Read the model definition and answer for the solid it produces. Units are mm, in the model's axes. A direction names the side the tool comes from. Give positions to 0.01 mm unless a question says otherwise; leave off trailing zeros.
Item 1: A cutting plane is placed at A-A (z = 43). State how many separate pieces and enclosed holes the cut face has, plus the area to 3 significant figures.
Item 2: Given pin 1 Ø1 at (x, z) = (0.5, 168.5) entering from +Y; pin 2 Ø0.6 at (x, z) = (-3, 123.5) entering from +Y, each flat-ended and moving along its own axis, determine where each tip first touches the part or whether it passes through.
Item 3: Which of the six approach directions +Z, -Z, +X, -X, +Y, -Y give full straight-line access (tool end or side, diameter ignored) to faces 1 (the face through (0, 4.5, 148)), 2 (the face through (-10, -6, 148))?
Item 4: Find the intervals of material crossed by line 1 along Y through (x, z) = (2.25, 271.5); line 2 along X through (y, z) = (0, 269.5); line 3 along Y through (x, z) = (2, 285.5), in increasing order.
Item 5: The mould has two halves that part along Y. Classify faces 3 (the face through (0, -8.5, 148)), 4 (the face through (4, 0, 0)), 5 (the face through (0, -10, 148)): +Y half, -Y half, draft (parallel to the pull), parting line (faces both ways), or undercut.
from build123d import *

# Parameters (mm, degrees)
BOSS_EXTRUDE1_DEPTH = 1000
CUT_EXTRUDE1_DEPTH  = 700


with BuildPart() as part:
    # Sketch1 → Boss-Extrude1 (new body)
    with BuildSketch(Plane.XY):
        with BuildLine():
            Line((6, 7.06066017), (3.43933983, 4.5))
            Line((3.43933983, 4.5), (-3.43933983, 4.5))
            Line((-3.43933983, 4.5), (-6, 7.06066017))
            Line((-6, 7.06066017), (-6, 8.5))
            Line((-6, 8.5), (-3, 8.5))
            Line((-3, 8.5), (-3, 9.5))
            Line((-3, 9.5), (-3.5, 9.5))
            Line((-3.5, 9.5), (-3.5, 10))
            Line((-3.5, 10), (-8.5, 10))
            ThreePointArc((-8.5, 10), (-9.56066017, 9.56066017), (-10, 8.5))
            Line((-10, 8.5), (-10, 3.5))
            Line((-10, 3.5), (-9.5, 3.5))
            Line((-9.5, 3.5), (-9.5, 3))
            Line((-9.5, 3), (-8.5, 3))
            Line((-8.5, 3), (-8.5, 6))
            Line((-8.5, 6), (-7.06066017, 6))
            Line((-7.06066017, 6), (-4.5, 3.43933983))
            Line((-4.5, 3.43933983), (-4.5, -3.43933983))
            Line((-4.5, -3.43933983), (-7.06066017, -6))
            Line((-7.06066017, -6), (-8.5, -6))
            Line((-8.5, -6), (-8.5, -3))
            Line((-8.5, -3), (-9.5, -3))
            Line((-9.5, -3), (-9.5, -3.5))
            Line((-9.5, -3.5), (-10, -3.5))
            Line((-10, -3.5), (-10, -8.5))
            ThreePointArc((-10, -8.5), (-9.56066017, -9.56066017), (-8.5, -10))
            Line((-8.5, -10), (8.5, -10))
            ThreePointArc((8.5, -10), (9.56066017, -9.56066017), (10, -8.5))
            Line((10, -8.5), (10, 8.5))
            ThreePointArc((10, 8.5), (9.56066017, 9.56066017), (8.5, 10))
            Line((8.5, 10), (3.5, 10))
            Line((3.5, 10), (3.5, 9.5))
            Line((3.5, 9.5), (3, 9.5))
            Line((3, 9.5), (3, 8.5))
            Line((3, 8.5), (6, 8.5))
            Line((6, 8.5), (6, 7.06066017))
        make_face()
        Polygon((4.5, -3.43933983), (4.5, 3.43933983), (7.79289322, 6.73223305), (8.5, 6.73223305), (8.5, -6.73223305), (7.79289322, -6.73223305), align=None, mode=Mode.SUBTRACT)
        with BuildLine():
            Line((-2.43563636, 1.27678327), (-3.0001742, 1.94957327))
            Line((-3.0001742, 1.94957327), (-1.94957327, 3.0001742))
            Line((-1.94957327, 3.0001742), (-1.27678327, 2.43563636))
            ThreePointArc((-1.27678327, 2.43563636), (0, 2.75), (1.27678327, 2.43563636))
            Line((1.27678327, 2.43563636), (1.94957327, 3.0001742))
            Line((1.94957327, 3.0001742), (3.0001742, 1.94957327))
            Line((3.0001742, 1.94957327), (2.43563636, 1.27678327))
            ThreePointArc((2.43563636, 1.27678327), (2.75, 0), (2.43563636, -1.27678327))
            Line((2.43563636, -1.27678327), (3.0001742, -1.94957327))
            Line((3.0001742, -1.94957327), (1.94957327, -3.0001742))
            Line((1.94957327, -3.0001742), (1.27678327, -2.43563636))
            ThreePointArc((1.27678327, -2.43563636), (0, -2.75), (-1.27678327, -2.43563636))
            Line((-1.27678327, -2.43563636), (-1.94957327, -3.0001742))
            Line((-1.94957327, -3.0001742), (-3.0001742, -1.94957327))
            Line((-3.0001742, -1.94957327), (-2.43563636, -1.27678327))
            ThreePointArc((-2.43563636, -1.27678327), (-2.75, 0), (-2.43563636, 1.27678327))
        make_face(mode=Mode.SUBTRACT)
        Polygon((3.43933983, -4.5), (6.73223305, -7.79289322), (6.73223305, -8.5), (-6.73223305, -8.5), (-6.73223305, -7.79289322), (-3.43933983, -4.5), align=None, mode=Mode.SUBTRACT)
    extrude(amount=BOSS_EXTRUDE1_DEPTH)

    # Sketch3 → Cut-Extrude1 (cut)
    with BuildSketch(Plane.XY.offset(1000)):
        with BuildLine():
            Line((6, 8.5), (6, 7.06066017))
            Line((6, 7.06066017), (3.43933983, 4.5))
            Line((3.43933983, 4.5), (-3.43933983, 4.5))
            Line((-3.43933983, 4.5), (-6, 7.06066017))
            Line((-6, 7.06066017), (-6, 8.5))
            Line((-6, 8.5), (-3, 8.5))
            Line((-3, 8.5), (-3, 9.5))
            Line((-3, 9.5), (-3.5, 9.5))
            Line((-3.5, 9.5), (-3.5, 10))
            Line((-3.5, 10), (-8.5, 10))
            ThreePointArc((-8.5, 10), (-9.56066017, 9.56066017), (-10, 8.5))
            Line((-10, 8.5), (-10, 3.5))
            Line((-10, 3.5), (-9.5, 3.5))
            Line((-9.5, 3.5), (-9.5, 3))
            Line((-9.5, 3), (-8.5, 3))
            Line((-8.5, 3), (-8.5, 6))
            Line((-8.5, 6), (-7.06066017, 6))
            Line((-7.06066017, 6), (-4.5, 3.43933983))
            Line((-4.5, 3.43933983), (-4.5, -3.43933983))
            Line((-4.5, -3.43933983), (-7.06066017, -6))
            Line((-7.06066017, -6), (-8.5, -6))
            Line((-8.5, -6), (-8.5, -3))
            Line((-8.5, -3), (-9.5, -3))
            Line((-9.5, -3), (-9.5, -3.5))
            Line((-9.5, -3.5), (-10, -3.5))
            Line((-10, -3.5), (-10, -8.5))
            ThreePointArc((-10, -8.5), (-9.56066017, -9.56066017), (-8.5, -10))
            Line((-8.5, -10), (8.5, -10))
            ThreePointArc((8.5, -10), (9.56066017, -9.56066017), (10, -8.5))
            Line((10, -8.5), (10, 8.5))
            ThreePointArc((10, 8.5), (9.56066017, 9.56066017), (8.5, 10))
            Line((8.5, 10), (3.5, 10))
            Line((3.5, 10), (3.5, 9.5))
            Line((3.5, 9.5), (3, 9.5))
            Line((3, 9.5), (3, 8.5))
            Line((3, 8.5), (6, 8.5))
        make_face()
    extrude(amount=-CUT_EXTRUDE1_DEPTH, mode=Mode.SUBTRACT)


solid = part.part
Response values:
1. separate pieces: 1
1. enclosed holes: 3
1. area: 181 mm2
2. pin 1: stops at y = 4.5
2. pin 2: stops at y = 9.5
3. face 1: +Z, -Z
3. face 2: +Z, -Z, -X, +Y, -Y
4. line 1: y = -10 to -8.5, -4.5 to -2.7, 2.7 to 4.5
4. line 2: x = -4.5 to -2.75, 2.75 to 4.5, 8.5 to 10
4. line 3: y = -10 to -8.5, -4.5 to -2.95, 2.95 to 4.5
5. face 3: undercut
5. face 4: draft
5. face 5: -Y half
